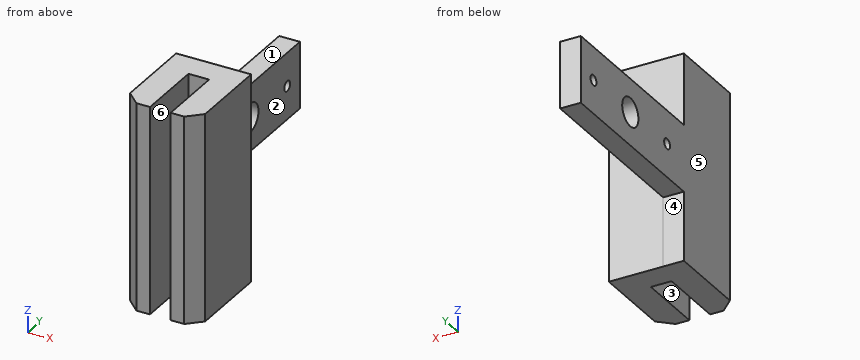
```python
from build123d import *

# Parameters (mm, degrees)
F1_DEPTH = 80
F2_R     = 2
F2_R_2   = 5.5
F3_DEPTH = 25


with BuildPart() as f1:
    # F0 (on Top) → F1 (new body)
    with BuildSketch(Plane.XY):
        Polygon((-14.5, 88.131121), (-14.5, 18.131121), (-14.5, -13.131121), (-9.25, -18.109524), (-4, -18.087926), (-4, 8.054228), (4, 8.054228), (4, -18.087926), (9.25, -18.109524), (14.5, -13.131121), (14.5, 18.131121), (-6.5, 18.131121), (-6.5, 88.131121), align=None)
    extrude(amount=F1_DEPTH)

    # F2 (on Right) → F3 (cut)
    with BuildSketch(Plane.YZ):
        Polygon((23.512104, 52.394919), (88.131121, 52.394919), (88.131121, 80), (18.131121, 80), (18.131121, 52.394919), align=None)
        Polygon((88.131121, -0.940287), (88.131121, 26.664793), (23.512104, 26.664793), (19.000409, 26.664793), (18.146811, 26.664793), (18.146811, 0), (18.146811, -0.940287), align=None)
        with Locations((79.512104, 39.529856)):
            Circle(F2_R)
        with Locations((54.512104, 39.529856)):
            Circle(F2_R_2)
        with Locations((29.512104, 39.529856)):
            Circle(F2_R)
    extrude(amount=-F3_DEPTH, mode=Mode.SUBTRACT)


solid = f1.part
```
The listing builds one solid part. Answer for the finished solid, in the listing's coordinates (mm). Face numbers are marked on the shaded views. A direction names the side the tool comes from. Coordinates: 2 decimals unless noted, no trailing zeros. Loops run counter-clockwise (first coordinate to the right, second up) from the corner with the lowest first, then second, coordinate; pieces in that order, holes last. Notation, with made-up numbers: (88.5, -15) - (134.5, -15) arc R10 ccw to (134.5, -8) - close; hole circle Ø1 at (27, 10.25). An arc over 180 degrees is marked (long way). Write item = value, one per line.
1) Determine the mould class of the marked faces 4, 5 and 6 for opening direction X: pulls with the +X half, pulls with the -X half, needs draft (parallel to the pull), parting line crosses it, or undercut.
Responses:
face_4 = needs draft
face_5 = pulls with the -X half
face_6 = undercut
2) Section D-D (z = 32.5) is taken. Determine the outline of the cut face in (x, y).
Responses:
outline = (-14.5, -13.13) - (-9.25, -18.11) - (-4, -18.09) - (-4, 8.05) - (4, 8.05) - (4, -18.09) - (9.25, -18.11) - (14.5, -13.13) - (14.5, 18.13) - (-6.5, 18.13) - (-6.5, 88.13) - (-14.5, 88.13) - close
3) Section C-C (y = 79) is taken. Determine the outline of the cut face in (x, z).
Responses:
outline = (-14.5, 26.66) - (-6.5, 26.66) - (-6.5, 37.6) - (-14.5, 37.6) - close; (-14.5, 41.46) - (-6.5, 41.46) - (-6.5, 52.39) - (-14.5, 52.39) - close
4) Each of these flat-tipped pins is pushed along its axis until it touches: P1, Ø2.5, axis at x = -9.5, z = 12.5, coming from the +Y side; P2, Ø6.5, axis at y = 29.51, z = 39.53, coming from the -X side; P3, Ø3, axis at x = 3.5, z = 43, coming from the -Y side; P4, Ø2, axis at x = -9.5, y = 59, coming from the -Z side. Where does it stop, or does it pass through?
Responses:
P1 = 18.15
P2 = -14.5
P3 = -18.09
P4 = 26.66
5) Find the intervals of material crossed by line 1 along X through (y, z) = (6, 39); line 2 along Z through (x, y) = (-10.75, 36); line 3 along Y through (x, z) = (3, 38), in increasing order.
Responses:
line_1 = -14.5 to -4, 4 to 14.5
line_2 = 26.66 to 52.39
line_3 = 8.05 to 18.13
6) Section B-B (z = 67.5) is taken. Determine the outline of the cut face in (x, y).
Responses:
outline = (-14.5, -13.13) - (-9.25, -18.11) - (-4, -18.09) - (-4, 8.05) - (4, 8.05) - (4, -18.09) - (9.25, -18.11) - (14.5, -13.13) - (14.5, 18.13) - (-14.5, 18.13) - close
7) Which of the six approach directions +Z, -Z, +X, -X, +Y, -Y give full straight-line access (tool end or side, diameter ignored) to the marked faces 1, 2 and 3?
Responses:
face_1 = +Z, +X, -X, +Y
face_2 = +Z, -Z, +X, +Y
face_3 = +Z, -Z, -Y
8) Section A-A (y = 55.5) is taken. Determine the outline of the cut face in (x, z), plus the area to 3 significant figures.
Responses:
outline = (-14.5, 26.66) - (-6.5, 26.66) - (-6.5, 34.12) - (-14.5, 34.12) - close; (-14.5, 44.94) - (-6.5, 44.94) - (-6.5, 52.39) - (-14.5, 52.39) - close
area = 119 mm^2
